For this review, take the finished solid that the model builds, in its own axes (mm). A direction names the side the tool comes from. Give positions to 0.01 mm unless a question says otherwise; leave off trailing zeros. Write each loop counter-clockwise with the first axis right and the second up, starting at its lowest first coordinate (ties: lowest second). Pieces come first, ordered by that corner, then holes. Notation, with made-up numbers: (-21, 72) -> (-11, 72) arc R16 ccw to (-11, 94) -> close; hole circle Ø5 at (-10, 63). An arc over 180 degrees is marked (long way). Answer as CSV lines item,"result".
```python
from build123d import *

# Parameters (mm, degrees)
SKETCH_W        = 12
SKETCH_H        = 32
SKETCH_R        = 2.5
PAD_DEPTH       = 25
SKETCH001_R     = 6
POCKET_DEPTH    = 12
SKETCH002_R     = 5
POCKET001_DEPTH = 5


with BuildPart() as part:
    # Sketch → Pad (new body)
    with BuildSketch(Plane.XZ):
        Rectangle(SKETCH_W, SKETCH_H)
        with Locations((0, 8.5)):
            Circle(SKETCH_R, mode=Mode.SUBTRACT)
        with Locations((0, -8.5)):
            Circle(SKETCH_R, mode=Mode.SUBTRACT)
    extrude(amount=PAD_DEPTH)

    # Sketch001 → Pocket (cut)
    with BuildSketch(Plane(origin=(-6, 0, 0), x_dir=(0, 0, -1), z_dir=(-1, 0, 0))):
        with Locations((0, 12.5)):
            Circle(SKETCH001_R)
    extrude(amount=-POCKET_DEPTH, mode=Mode.SUBTRACT)

    # Sketch002 → Pocket001 (cut)
    with BuildSketch(Plane.XZ.offset(25)):
        with Locations((0, 8.5)):
            Circle(SKETCH002_R)
        with Locations((0, -8.5)):
            Circle(SKETCH002_R)
    extrude(amount=-POCKET001_DEPTH, mode=Mode.SUBTRACT)


solid = part.part
```
Q1. Draft analysis for pull direction X (two halves, no side actions). For faces 3 (the flat face through (0, 0, 0)), 4 (the cylindrical face through (-0.54, -9.86, -10.94)), 5 (the cylindrical face through (-0.651, -22.535, 13.457)), 6 (the flat face through (6, -7, -4)), state which applies: released by +X, released by -X, zero draft, split by the parting line, or undercut.
Answer block:
face 3,"zero draft"
face 4,"undercut"
face 5,"undercut"
face 6,"released by +X"
Q2. To check wall thickness, follow probe 1 along Z at (x, y) = (0, -21); probe 2 along X at (y, z) = (-9.5, -8.5); probe 3 along Z at (x, y) = (1.5, -12.5). State the ranges of each line that lie inside material, in increasing order. Write a range as [from, to].
Answer block:
probe 1,"z = [-16, -13.5], [-3.5, 3.5], [13.5, 16]"
probe 2,"x = [-6, -2.5], [2.5, 6]"
probe 3,"z = [-16, -10.5], [-6.5, -6], [6, 6.5], [10.5, 16]"
Q3. Clearance check with a flat-ended pin moving along its axis: pin 1 (6.5 mm diameter, centred on x = 0, z = 8.5, fed in from -Y). State where the tip first meets the part, or that it passes through.
Answer block:
pin 1,"stops at y = -20"
Q4. Add section D-D (y = -23). Write out the cut boundary in (x, z).
Answer block:
outline,"(-6, -16) -> (6, -16) -> (6, 16) -> (-6, 16) -> close; hole circle Ø10 at (0, -8.5); hole circle Ø10 at (0, 8.5)"
Q5. For faces 1 (the cylindrical face through (-0.54, -9.86, 6.06)), 2 (the flat face through (1, -20, -6)), list the 3-axis set-ups (+Z, -Z, +X, -X, +Y, -Y) from which the entire face can be reached by the end or side of a thin tool; tool diameter is ignored.
Answer block:
face 1,"+Y, -Y"
face 2,"-Y"
Q6. Add section B-B (z = 8.5). Write out the cut boundary in (x, y), plus the area to 3 significant figures.
Answer block:
outline,"(-6, -25) -> (-5, -25) -> (-5, -20) -> (-2.5, -20) -> (-2.5, 0) -> (-6, 0) -> close; (2.5, -20) -> (5, -20) -> (5, -25) -> (6, -25) -> (6, 0) -> (2.5, 0) -> close"
area,"150 mm2"
Q7. Add section C-C (x = -4). Write out the cut boundary in (y, z), plus the area to 3 significant figures.
Answer block:
outline,"(-25, -16) -> (0, -16) -> (0, 16) -> (-25, 16) -> (-25, 11.5) -> (-20, 11.5) -> (-20, 5.5) -> (-25, 5.5) -> (-25, -5.5) -> (-20, -5.5) -> (-20, -11.5) -> (-25, -11.5) -> close; hole circle Ø12 at (-12.5, 0)"
area,"627 mm2"
Q8. Add section A-A (y = -12.5). Write out the cut boundary in (x, z).
Answer block:
outline,"(-6, -16) -> (6, -16) -> (6, -6) -> (-6, -6) -> close; (-6, 6) -> (6, 6) -> (6, 16) -> (-6, 16) -> close; hole circle Ø5 at (0, -8.5); hole circle Ø5 at (0, 8.5)"
